For this review, take the finished solid that the model builds, in its own axes (mm). A direction names the side the tool comes from. Coordinates: 2 decimals unless noted, no trailing zeros. Write each loop counter-clockwise with the first axis right and the second up, starting at its lowest first coordinate (ties: lowest second). Pieces come first, ordered by that corner, then holes.
1) For faces 1 (the face through (48, -1.596, 9)), 2 (the face through (48, -9, -1.593)), 3 (the face through (48, 1.579, 9)), list the 3-axis set-ups (+Z, -Z, +X, -X, +Y, -Y) from which the entire face can be reached by the end or side of a thin tool; tool diameter is ignored.
2) To check wall thickness, follow line 1 along X through (y, z) = (1.25, 14); line 2 along Y through (x, z) = (50, 13.5); line 3 along Z through (x, y) = (19, 0.25). State the ranges of each line that lie inside material, in increasing order.
3) We need section C-C on x = 35. Write out the cut boundary in (y, z) (3 decimals).
4) We need section D-D on z = 10.5. Write out the cut boundary in (x, y), then the cut area to 3 significant figures.
5) We need section A-A on z = 0. Write out the cut boundary in (x, y) (3 decimals), then the cut area to 3 significant figures.
6) Insertion check: P1, Ø4, axis at y = -3.5, z = 8, coming from the +X side; P2, Ø2.5, axis at y = 0.5, z = 7.5, coming from the -X side; P3, Ø5, axis at x = 48, y = -7.5, coming from the -Z side; P4, Ø1.5, axis at x = 57.5, z = 5, coming from the +Y side. Each pin has a flat end and moves straight along its axis. Give the tip position at first contact, or say it passes through.
from build123d import *

# Parameters (mm, degrees)
F0_R     = 3.175
F1_DEPTH = 114.3
F5_DEPTH = 6.35


with BuildPart() as f1:
    # F0 (on Right) → F1 (new body)
    with BuildSketch(Plane.YZ):
        Circle(F0_R)
    extrude(amount=F1_DEPTH)

    # F4 (on offset) → F5 (join)
    with BuildSketch(Plane(origin=(44.45, 0, 0), x_dir=(0, -1, 0), z_dir=(-1, 0, 0))):
        with BuildLine():
            Line((15.4581812469, 1.5823668619), (2.7581812469, 1.5823668619))
            Line((2.7581812469, 1.5823668619), (2.7581812469, 1.571402878))
            ThreePointArc((2.7581812469, 1.571402878), (3.0685880653, 0.8127964573), (3.1744087316, 0))
            ThreePointArc((3.1744087316, 0), (3.0685880653, -0.8127964573), (2.7581812469, -1.571402878))
            Line((2.7581812469, -1.571402878), (2.7581812469, -1.5926331381))
            Line((2.7581812469, -1.5926331381), (15.4581812469, -1.5926331381))
            Line((15.4581812469, -1.5926331381), (15.4581812469, 1.5823668619))
        make_face()
        with BuildLine():
            ThreePointArc((-1.5789494102, 2.7538681079), (0.0093713682, 3.1743948987), (1.5951815458, 2.7444975189))
            Line((1.5951815458, 2.7444975189), (1.5960505898, 2.7444975189))
            Line((1.5960505898, 2.7444975189), (1.5960505898, 15.4444975189))
            Line((1.5960505898, 15.4444975189), (-1.5789494102, 15.4444975189))
            Line((-1.5789494102, 15.4444975189), (-1.5789494102, 2.7538681079))
        make_face()
    extrude(amount=-F5_DEPTH)


solid = f1.part
Result:
1. face 1: +Z, +X, -X, -Y
1. face 2: -Z, +X, -X, -Y
1. face 3: +Z, +X, -X, +Y
2. line 1: x = 44.45 to 50.8
2. line 2: y = -1.6 to 1.58
2. line 3: z = -3.17 to 3.17
3. outline: circle Ø6.35 at (0, 0)
4. outline: (44.45, -1.6) - (50.8, -1.6) - (50.8, 1.58) - (44.45, 1.58) - close
4. area: 20.2 mm2
5. outline: (0, -3.175) - (44.45, -3.175) - (44.45, -15.458) - (50.8, -15.458) - (50.8, -3.175) - (114.3, -3.175) - (114.3, 3.175) - (0, 3.175) - close
5. area: 804 mm2
6. P1: stops at x = 50.8
6. P2: stops at x = 44.45
6. P3: stops at z = -1.59
6. P4: passes through
